The figure shows three views and two pictorial views of one solid part (mm, origin at its lowest corner). Answer the questions. A direction names the side the tool comes from. Round coordinates to 2 decimals unless told otherwise and drop trailing zeros. Order: outer loops, then holes, each group sorted by start corner. A loop starts at its lowest first (then second) coordinate and runs counter-clockwise, first axis right, second up. Notation, with made-up numbers: (-21.75, 52.5) - (12.25, 52.5) arc R21 ccw to (12.25, 63.5) - close; hole circle Ø11 at (25.25, -38.75). An arc over 180 degrees is marked (long way). Answer in a Markdown table with one row per item.
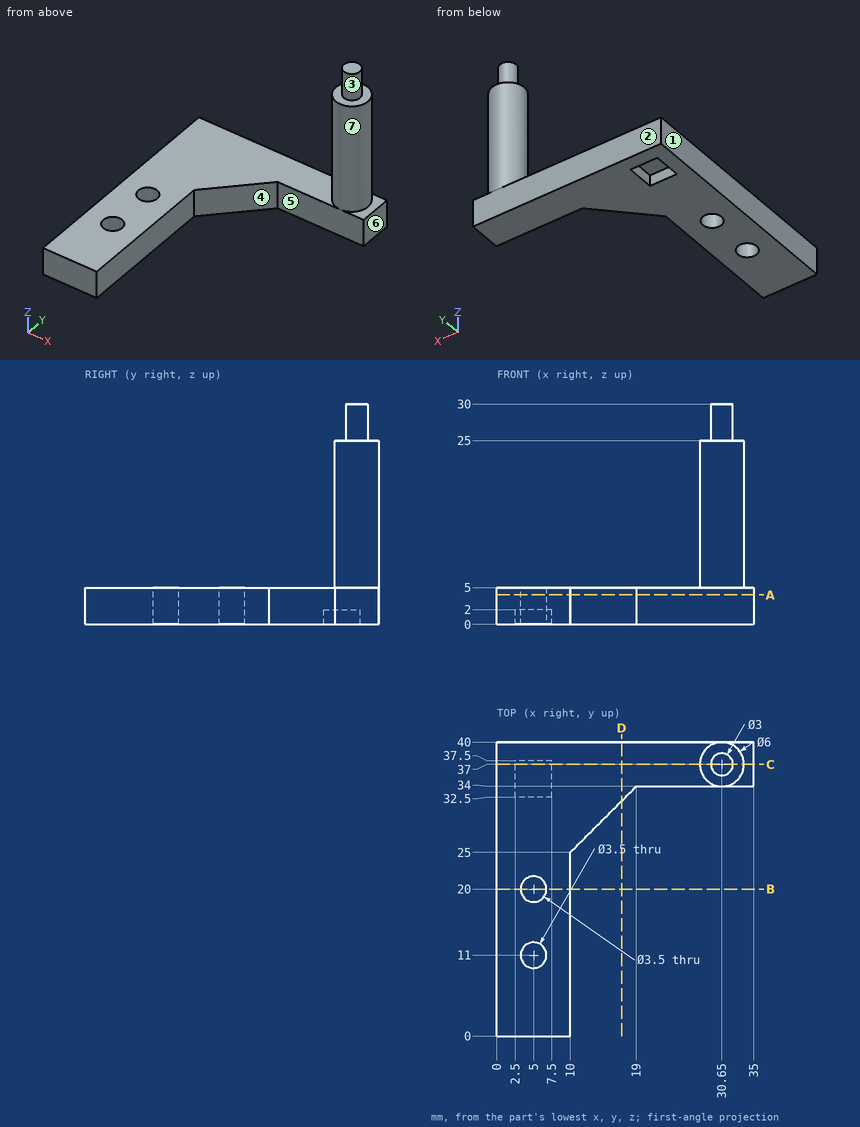
1) Find section D-D, the plane x = 17. Give the vertices of the cut face in (y, z).
Filled in:
| item | result |
|---|---|
| outline | (32, 0) - (40, 0) - (40, 5) - (32, 5) - close |
2) Each of these flat-tipped pins is pushed along its axis until it touches: pin 1 (8 mm diameter, centred on x = 30.5, z = 17, fed in from -Y); pin 2 (15.5 mm diameter, centred on x = 15.5, y = 10.5, fed in from +Z); pin 3 (1.5 mm diameter, centred on y = 16.5, z = 1.5, fed in from +X). Where does it stop, or does it pass through?
Filled in:
| item | result |
|---|---|
| pin 1 | stops at y = 34 |
| pin 2 | stops at z = 5 |
| pin 3 | stops at x = 10 |
3) Find section B-B, the plane y = 20. Give the vertices of the cut face in (x, z).
Filled in:
| item | result |
|---|---|
| outline | (0, 0) - (3.25, 0) - (3.25, 5) - (0, 5) - close; (6.75, 0) - (10, 0) - (10, 5) - (6.75, 5) - close |
4) The mould has two halves that part along Y. Classify the marked faces 1, 2, 3 and 4: released by +Y, released by -Y, zero draft, split by the parting line, or undercut.
Filled in:
| item | result |
|---|---|
| face 1 | zero draft |
| face 2 | released by +Y |
| face 3 | split by the parting line |
| face 4 | released by -Y |
5) Which of the six approach directions +Z, -Z, +X, -X, +Y, -Y give full straight-line access (tool end or side, diameter ignored) to the marked faces 5, 6 and 7?
Filled in:
| item | result |
|---|---|
| face 5 | +Z, -Z, +X, -Y |
| face 6 | +Z, -Z, +X, +Y, -Y |
| face 7 | +Z |
6) Find the intervals of material crossed by probe 1 along Y at (x, z) = (5, 3.5); probe 2 along Y at (x, z) = (5, 1.8); probe 3 along Z at (x, y) = (6, 29.5), in increasing order. Write a range as from..to.
Filled in:
| item | result |
|---|---|
| probe 1 | y = 0..9.25, 12.75..18.25, 21.75..40 |
| probe 2 | y = 0..9.25, 12.75..18.25, 21.75..32.5, 37.5..40 |
| probe 3 | z = 0..5 |
7) Find section A-A, the plane z = 4. Give the vertices of the cut face in (x, y).
Filled in:
| item | result |
|---|---|
| outline | (0, 0) - (10, 0) - (10, 25) - (19, 34) - (35, 34) - (35, 40) - (0, 40) - close; hole circle Ø3.5 at (5, 11); hole circle Ø3.5 at (5, 20) |
8) Find section C-C, the plane y = 37. Give the vertices of the cut face in (x, z).
Filled in:
| item | result |
|---|---|
| outline | (0, 0) - (2.5, 0) - (2.5, 2) - (7.5, 2) - (7.5, 0) - (35, 0) - (35, 5) - (33.65, 5) - (33.65, 25) - (32.15, 25) - (32.15, 30) - (29.15, 30) - (29.15, 25) - (27.65, 25) - (27.65, 5) - (0, 5) - close |
